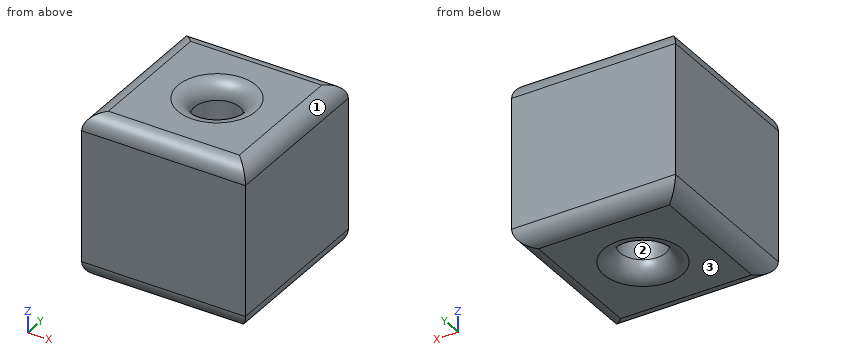
```python
from build123d import *

# Parameters (mm, degrees)
F0_W     = 50
F0_H     = 50
F0_R     = 6.92614
F1_DEPTH = 50
F2_DEPTH = 20
F3_R     = 5
F4_R     = 5


with BuildPart() as f1:
    # F0 (on Top) → F1 (new body)
    with BuildSketch(Plane.XY):
        with Locations((-0.460617, -0.251955)):
            Rectangle(F0_W, F0_H)
        Circle(F0_R, mode=Mode.SUBTRACT)
    extrude(amount=F1_DEPTH)

    # F0 (on Top) → F2 (cut)
    with BuildSketch(Plane.XY):
        with Locations((-0.460617, -0.251955)):
            Rectangle(F0_W, F0_H)
        Circle(F0_R, mode=Mode.SUBTRACT)
    extrude(amount=-F2_DEPTH, mode=Mode.SUBTRACT)

    # F3
    f3_edges = [f1.edges().sort_by_distance(p)[0] for p in [
        (-0.460617, 24.748045, 50),
        (-25.460617, -0.251955, 50),
        (-0.460617, -25.251955, 50),
        (24.539383, -0.251955, 50),
        (-6.92614, 0, 50),
    ]]
    fillet(f3_edges, radius=F3_R)

    # F4
    f4_edges = [f1.edges().sort_by_distance(p)[0] for p in [
        (-0.460617, 24.748045, 0),
        (-25.460617, -0.251955, 0),
        (-0.460617, -25.251955, 0),
        (24.539383, -0.251955, 0),
        (-6.92614, 0, 0),
    ]]
    fillet(f4_edges, radius=F4_R)


solid = f1.part
```
Part model, mm, in its own coordinate system. Face numbers are marked on the shaded views. Round coordinates to 2 decimals unless told otherwise and drop trailing zeros. Write each loop counter-clockwise with the first axis right and the second up, starting at its lowest first coordinate (ties: lowest second). Pieces come first, ordered by that corner, then holes.
Item 1: Probe L1, parallel to Y at x = 0, z = 15; L2, parallel to X at y = -1, z = 36; L3, parallel to Z at x = 20, y = -22.5. List the from-to ranges inside material, lowest first.
Results:
L1: y = -25.25 to -6.93, 6.93 to 24.75
L2: x = -25.46 to -6.85, 6.85 to 24.54
L3: z = 0.53 to 49.47
Item 2: Cut at A-A, the plane y = 0. Give the cut face in (x, z), plus the area to 3 significant figures.
Results:
outline: (-25.46, 5) arc R5 ccw to (-20.46, 0) - (-11.93, 0) arc R5 ccw to (-6.93, 5) - (-6.93, 45) arc R5 ccw to (-11.93, 50) - (-20.46, 50) arc R5 ccw to (-25.46, 45) - close; (6.93, 5) arc R5 ccw to (11.93, 0) - (19.54, 0) arc R5 ccw to (24.54, 5) - (24.54, 45) arc R5 ccw to (19.54, 50) - (11.93, 50) arc R5 ccw to (6.93, 45) - close
area: 1,760 mm2
Item 3: Two-plate mould, pull along X, no slides. Class the marked faces 1, 2 and 3: +X half, -X half, draft (parallel to the pull), parting line (faces both ways), or undercut.
Results:
face 1: +X half
face 2: undercut
face 3: draft
Item 4: Cut at B-B, the plane x = 0. Give the cut face in (y, z), plus the area to 3 significant figures.
Results:
outline: (-25.25, 5) arc R5 ccw to (-20.25, 0) - (-11.93, 0) arc R5 ccw to (-6.93, 5) - (-6.93, 45) arc R5 ccw to (-11.93, 50) - (-20.25, 50) arc R5 ccw to (-25.25, 45) - close; (6.93, 5) arc R5 ccw to (11.93, 0) - (19.75, 0) arc R5 ccw to (24.75, 5) - (24.75, 45) arc R5 ccw to (19.75, 50) - (11.93, 50) arc R5 ccw to (6.93, 45) - close
area: 1,760 mm2
Item 5: Cut at C-C, the plane z = 13.5. Give the cut face in (x, y), plus the area to 3 significant figures.
Results:
outline: (-25.46, -25.25) - (24.54, -25.25) - (24.54, 24.75) - (-25.46, 24.75) - close; hole circle Ø13.85 at (0, 0)
area: 2,350 mm2
Item 6: Drop flat-ended pins along their axis: pin 1 Ø18 at (x, y) = (0, 0) entering from +Z; pin 2 Ø6 at (x, y) = (3.5, 8) entering from -Z; pin 3 Ø2 at (x, y) = (-2.5, -6.5) entering from +Z; pin 4 Ø5 at (x, y) = (2.5, 2) entering from +Z. Give the stop position or say it passes through.
Results:
pin 1: stops at z = 49.05
pin 2: stops at z = 0
pin 3: stops at z = 48.05
pin 4: passes through
